```python
from build123d import *

# Parameters (mm, degrees)
EXTRUDE_1_DEPTH     = 20
SKETCH_8_W          = 4
SKETCH_8_H          = 32
SKETCH_11_W         = 4
SKETCH_11_H         = 32
SKETCH_13_R         = 16
CUT_EXTRUDE_4_DEPTH = 202.639119047
SKETCH_16_R         = 16
EXTRUDE_4_DEPTH     = 8
SKETCH_17_W         = 276.65605666
SKETCH_17_H         = 73.661463051
CUT_EXTRUDE_5_DEPTH = 234.318180858


with BuildPart() as part:
    # 草图2 → 凸台-拉伸1 (new body)
    with BuildSketch(Plane(origin=(0, 0, 0), x_dir=(1, 0, 0), z_dir=(0, 1, 0))):
        with BuildLine():
            Line((-40, 84), (40, 84))
            ThreePointArc((40, 84), (124, 0), (40, -84))
            Line((40, -84), (-40, -84))
            ThreePointArc((-40, -84), (-124, 0), (-40, 84))
        make_face()
        with BuildLine():
            Line((-40, 80), (40, 80))
            ThreePointArc((40, 80), (120, 0), (40, -80))
            Line((40, -80), (-40, -80))
            ThreePointArc((-40, -80), (-120, 0), (-40, 80))
        make_face(mode=Mode.SUBTRACT)
    extrude(amount=EXTRUDE_1_DEPTH)

    # 扫描1: sweep along a path in 草图9
    with BuildLine(Plane.XY) as sweep_1_path:
        Line((-124, 20), (-124, 0))
        Line((-124, 0), (-155, -80))
    # 草图8 → 扫描1 (sweep)
    with BuildSketch(Plane(origin=(0, 20, 0), x_dir=(1, 0, 0), z_dir=(0, 1, 0))):
        with Locations((-122, 0)):
            Rectangle(SKETCH_8_W, SKETCH_8_H)
    sweep(path=sweep_1_path.line, transition=Transition.RIGHT)

    # 扫描2: sweep along a path in 草图12
    with BuildLine(Plane.XY) as sweep_2_path:
        Line((124, 20), (124, 0))
        Line((124, 0), (155, -80))
    # 草图11 → 扫描2 (sweep)
    with BuildSketch(Plane(origin=(0, 20, 0), x_dir=(1, 0, 0), z_dir=(0, 1, 0))):
        with Locations((122, 0)):
            Rectangle(SKETCH_11_W, SKETCH_11_H)
    sweep(path=sweep_2_path.line, transition=Transition.RIGHT)

    # 草图13 → 切除-拉伸4 (cut, through all)
    with BuildSketch(Plane.XY.offset(16)):
        with Locations((-167.270234139, -81.445284271)):
            Circle(SKETCH_13_R)
        with Locations((167.270234139, -81.445284271)):
            Circle(SKETCH_13_R)
    extrude(amount=-CUT_EXTRUDE_4_DEPTH, mode=Mode.SUBTRACT)

    # 草图16 → 凸台-拉伸4 (add, symmetric)
    with BuildSketch(Plane.XY):
        with Locations((167.270234139, -81.445284271)):
            Circle(SKETCH_16_R)
        with Locations((-167.270234139, -81.445284271)):
            Circle(SKETCH_16_R)
    extrude(amount=EXTRUDE_4_DEPTH, both=True)

    # 草图17 → 切除-拉伸5 (cut, through all)
    with BuildSketch(Plane(origin=(0, 20, 0), x_dir=(1, 0, 0), z_dir=(0, 1, 0))):
        with Locations((14.32802833, -52.830731526)):
            Rectangle(SKETCH_17_W, SKETCH_17_H)
    extrude(amount=-CUT_EXTRUDE_5_DEPTH, mode=Mode.SUBTRACT)


solid = part.part
```
Verification items for the finished model (mm, model axes). A direction names the side the tool comes from. Coordinates: 2 decimals unless noted, no trailing zeros. Write each loop counter-clockwise with the first axis right and the second up, starting at its lowest first coordinate (ties: lowest second). Pieces come first, ordered by that corner, then holes. Notation, with made-up numbers: M 71,17.25 L 104,17.25 A20 cw 104,55.25 Z; hole C -23.5,-7.75 d1. An arc over 180 degrees is marked long. One line per item, written item: value.
Item 1: Gauge pin test, flat ends, axial feed: pin 1 Ø9.5 at (x, y) = (174.5, -79) entering from -Z; pin 2 Ø6 at (y, z) = (-13.5, -4.5) entering from +X; pin 3 Ø0.5 at (x, z) = (-119.5, 7) entering from -Y. Record the tip position at first contact, or that the pin passes through.
Check sheet entries:
pin 1: stops at z = -8
pin 2: stops at x = 130.39
pin 3: stops at y = 0
Item 2: Mould release check, pull along X, two halves, no side actions. Record for faces 5 (the cylindrical face through (182.708, -85.649, 0.112)), 6 (the flat face through (-130, -24, 16)), 7 (the cylindrical face through (92.813, 9.86, -65.32)): pulls with the +X half, pulls with the -X half, needs draft (parallel to the pull), parting line crosses it, or undercut.
Check sheet entries:
face 5: undercut
face 6: needs draft
face 7: pulls with the +X half
Item 3: Section check B-B, the plane y = -31.5. Record the boundary of the cut face in (x, z), plus the area to 3 significant figures.
Check sheet entries:
outline: M -136.21,-16 L -131.92,-16 L -131.92,16 L -136.21,16 Z; M 131.92,-16 L 136.21,-16 L 136.21,16 L 131.92,16 Z
area: 275 mm^2
Item 4: Section check A-A, the plane z = -3.5. Record the boundary of the cut face in (x, y), plus the area to 3 significant figures.
Check sheet entries:
outline: M -152.86,-74.49 A16 ccw long -151.27,-81.45 L -120,-0.75 L -120,0 L -119.92,0 L -119.92,20 L -124,20 L -124,0 Z; M 119.92,0 L 120,0 L 120,-0.75 L 151.27,-81.45 A16 ccw long 152.86,-74.49 L 124,0 L 124,20 L 119.92,20 Z
area: 2,440 mm^2
Item 5: Scan lines: line 1 along Z through (x, y) = (-136, -38.5); line 2 along X through (y, z) = (13.5, -18); line 3 along X through (y, z) = (9.5, -69). Record each from-to range of solid material in increasing order.
Check sheet entries:
line 1: z = -16 to 16
line 2: x = -122.05 to -117.95, 117.95 to 122.05
line 3: x = -87.91 to -80.48, 80.48 to 87.91
Item 6: Section check C-C, the plane y = 13. Record the boundary of the cut face in (x, z).
Check sheet entries:
outline: M -124,-16 L -122.46,-16 A84 ccw -40,-84 L 40,-84 A84 ccw 122.46,-16 L 124,-16 L 124,16 L 118.38,16 A80 cw 40,-80 L -40,-80 A80 cw -118.38,16 L -124,16 Z
Item 7: Access from +Z, -Z, +X, -X, +Y, -Y to the whole of each face (thin tool, end or side, straight path). Record for faces 1 (the cylindrical face through (-102.591, 9.86, -49.824)), 2 (the flat face through (-124, 10, 0)), 3 (the cylindrical face through (-151.662, -77.925, -11.944)), 4 (the flat face through (124, 10, 0)).
Check sheet entries:
face 1: +Y, -Y
face 2: +Z, -Z, -X, +Y
face 3: -Z, -X, -Y
face 4: +Z, -Z, +X, +Y
Item 8: Section check D-D, the plane x = 10.5. Record the boundary of the cut face in (y, z), plus the area to 3 significant figures.
Check sheet entries:
outline: M 0,-84 L 20,-84 L 20,-80 L 0,-80 Z
area: 80.0 mm^2
